Design review of the part built by this model. Coordinates are the model's own, in mm. A direction names the side the tool comes from. Give positions to 0.01 mm unless a question says otherwise; leave off trailing zeros. Order: outer loops, then holes, each group sorted by start corner. A loop starts at its lowest first (then second) coordinate and runs counter-clockwise, first axis right, second up. Notation, with made-up numbers: (-33, -34.5) -> (0, -34.5) arc R20 cw to (0, -25.5) -> close; hole circle Ø4 at (60.25, 41.5). An arc over 180 degrees is marked (long way). One line per item, written item: value.
from build123d import *

# Parameters (mm, degrees)
SKETCH1_R      = 2.4585
BASENUT_DEPTH  = 3.92
EXTRUDE1_START = 4.08
SKETCH2_R      = 4.89
SKETCH2_R_2    = 2.4585
EXTRUDE1_DEPTH = 4.08
CHAMFER1_SIZE  = 0.1956


with BuildPart() as part:
    # Sketch1 → BaseNut (new body)
    with BuildSketch(Plane.XY):
        Polygon((2.886751346, -5), (5.773502692, 0), (2.886751346, 5), (-2.886751346, 5), (-5.773502692, 0), (-2.886751346, -5), align=None)
        Circle(SKETCH1_R, mode=Mode.SUBTRACT)
    extrude(amount=-BASENUT_DEPTH)

    # Sketch3 → Double-Chamfer (revolve, cut)
    with BuildSketch(Plane(origin=(0, 0, 0), x_dir=(1, 0, 0), z_dir=(0, 1, 0)), mode=Mode.PRIVATE) as double_chamfer_sk:
        Polygon((4.44, 3.92), (5.773502692, 3.92), (5.773502692, 3.150101862), align=None)
        Polygon((5.773502692, 0.769898138), (4.44, 0), (5.773502692, 0), align=None)
    revolve(double_chamfer_sk.sketch.rotate(Axis((0, 0, -16.31077227), (0, 0, 1)), 179.999999973), axis=Axis((0, 0, -16.31077227), (0, 0, 1)), mode=Mode.SUBTRACT)

    # Sketch2 → Extrude1 (add)
    with BuildSketch(Plane(origin=(20.087129569, -4.281493882, 0), x_dir=(1, 0, 0), z_dir=(0, 0, 1)).offset(EXTRUDE1_START)):
        with Locations((-20.087129569, 4.281493882)):
            Circle(SKETCH2_R)
        with Locations((-20.087129569, 4.281493882)):
            Circle(SKETCH2_R_2, mode=Mode.SUBTRACT)
    extrude(amount=-EXTRUDE1_DEPTH)

    # Sketch5 → EndChamfer (revolve, cut)
    with BuildSketch(Plane(origin=(0, 0, 0), x_dir=(1, 0, 0), z_dir=(0, 1, 0))):
        Polygon((2.4585, 3.92), (3.375, 3.92), (2.4585, 3.0035), align=None)
    revolve(axis=Axis((0, 0, -16.800797033), (0, 0, 1)), mode=Mode.SUBTRACT)

    # Chamfer1
    chamfer1_edges = [part.edges().sort_by_distance(p)[0] for p in [
        (-4.89, 0, 4.08),
    ]]
    chamfer(chamfer1_edges, length=CHAMFER1_SIZE)


solid = part.part
Item 1: To check wall thickness, follow line 1 along Y through (x, z) = (0, 0.5); line 2 along Z through (x, y) = (2.5, -1.75); line 3 along X through (y, z) = (1.75, 3.5). State the ranges of each line that lie inside material, in increasing order. Write a range as from..to.
Returned:
line 1: -4.89..-2.46, 2.46..4.89
line 2: -3.6..4.08
line 3: -4.57..-1.73, 1.73..4.57
Item 2: Clearance check with a flat-ended pin moving along its axis: P1, Ø4, axis at y = -3.5, z = -2.5, coming from the +X side. State where the tip first meets the part, or that it passes through.
Returned:
P1: x = 4.91
Item 3: Machinability: for faces 1 (the cylindrical face through (-1.06, -4.774, 1.969)), 2 (the cylindrical face through (2.345, 0.738, 0.588)), which of the approach directions +Z, -Z, +X, -X, +Y, -Y give a long, thin tool a straight path to every point of the face, cutting with its end or side? Answer none if there is none.
Returned:
face 1: +Z
face 2: +Z, -Z
Item 4: Add section C-C on z = 3.5. Give the boundary of the cut face in (x, y), plus the area to 3 significant figures.
Returned:
outline: circle Ø9.78 at (0, 0); hole circle Ø4.92 at (0, 0)
area: 56.1 mm²
Item 5: Add section A-A on z = -2.5. Give the boundary of the cut face in (x, y).
Returned:
outline: (-5.77, 0) -> (-2.89, -5) -> (2.89, -5) -> (5.77, 0) -> (2.89, 5) -> (-2.89, 5) -> close; hole circle Ø4.92 at (0, 0)
